Can you work these out from the model? Positions are in its coordinate system, mm. Face numbers are marked on the shaded views. A direction names the side the tool comes from. Give positions to 0.01 mm unless a question says otherwise; leave off trailing zeros. Write each loop counter-clockwise with the first axis right and the second up, starting at its lowest first coordinate (ties: lowest second). Pieces come first, ordered by that corner, then holes.
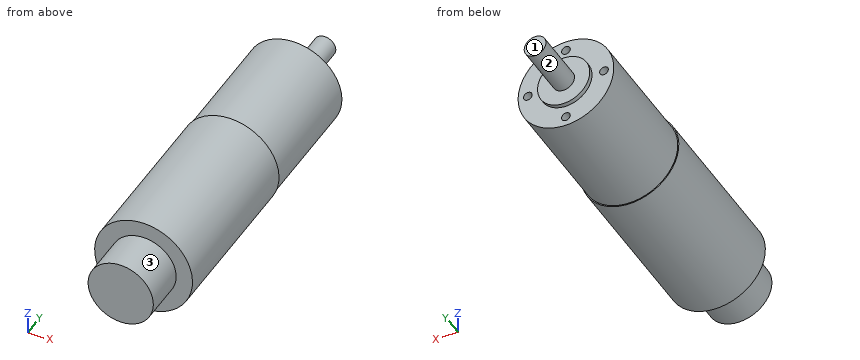
from build123d import *

# Parameters (mm, degrees)
SKETCH1_R           = 22.5
BOSS_EXTRUDE1_DEPTH = 75.7
SKETCH2_R           = 22
BOSS_EXTRUDE3_DEPTH = 56
SKETCH3_R           = 5
BOSS_EXTRUDE4_DEPTH = 27
SKETCH5_R           = 2
CUT_EXTRUDE2_DEPTH  = 9
CIRPATTERN1_COUNT   = 4
SKETCH6_R           = 12
BOSS_EXTRUDE5_DEPTH = 2
SKETCH7_R           = 15
BOSS_EXTRUDE6_DEPTH = 20


with BuildPart() as part:
    # Sketch1 → Boss-Extrude1 (new body)
    with BuildSketch(Plane(origin=(0, 0, 0), x_dir=(1, 0, 0), z_dir=(0, 1, 0))):
        with Locations(Location((0, 0, 0), (0, 0, 270))):
            Circle(SKETCH1_R)
    extrude(amount=BOSS_EXTRUDE1_DEPTH)

    # Sketch2 → Boss-Extrude3 (add)
    with BuildSketch(Plane(origin=(0, 75.7, 0), x_dir=(1, 0, 0), z_dir=(0, 1, 0))):
        with Locations(Location((0, 0, 0), (0, 0, 270))):
            Circle(SKETCH2_R)
    extrude(amount=BOSS_EXTRUDE3_DEPTH)

    # Sketch3 → Boss-Extrude4 (add)
    with BuildSketch(Plane(origin=(0, 131.7, 0), x_dir=(1, 0, 0), z_dir=(0, 1, 0))):
        with Locations(Location((0, 0, 0), (0, 0, 270))):
            Circle(SKETCH3_R)
    extrude(amount=BOSS_EXTRUDE4_DEPTH)

    # Sketch5 → Cut-Extrude2 (cut)
    with BuildSketch(Plane(origin=(0, 131.7, 0), x_dir=(1, 0, 0), z_dir=(0, 1, 0))):
        with Locations(Location((0, 17.5, 0), (0, 0, 270))):
            Circle(SKETCH5_R)
    cut_extrude2 = extrude(amount=-CUT_EXTRUDE2_DEPTH, mode=Mode.SUBTRACT)

    # CirPattern1: Cut-Extrude2 ×4 about axis
    cirpattern1_axis = Axis((0, 0, 0), (0, 1, 0))
    for i in range(1, CIRPATTERN1_COUNT):
        add(cut_extrude2.rotate(cirpattern1_axis, i * 360 / CIRPATTERN1_COUNT), mode=Mode.SUBTRACT)

    # Sketch6 → Boss-Extrude5 (add)
    with BuildSketch(Plane(origin=(0, 131.7, 0), x_dir=(1, 0, 0), z_dir=(0, 1, 0))):
        with Locations(Location((0, 0, 0), (0, 0, 270))):
            Circle(SKETCH6_R)
    extrude(amount=BOSS_EXTRUDE5_DEPTH)

    # Sketch7 → Boss-Extrude6 (add)
    with BuildSketch(Plane.XZ):
        with Locations(Location((0, 0, 0), (0, 0, 270))):
            Circle(SKETCH7_R)
    extrude(amount=BOSS_EXTRUDE6_DEPTH)


solid = part.part
(1) Imagine slicing it at D-D, the plane x = -10. Write out the boundary of the cut face in (y, z).
Returned:
outline: (-20, -11.18) - (0, -11.18) - (0, -20.16) - (75.7, -20.16) - (75.7, -19.6) - (131.7, -19.6) - (131.7, -6.63) - (133.7, -6.63) - (133.7, 6.63) - (131.7, 6.63) - (131.7, 19.6) - (75.7, 19.6) - (75.7, 20.16) - (0, 20.16) - (0, 11.18) - (-20, 11.18) - close
(2) Imagine slicing it at B-B, the plane x = 0. Write out the boundary of the cut face in (y, z), plus the area to 3 significant figures.
Returned:
outline: (-20, -15) - (0, -15) - (0, -22.5) - (75.7, -22.5) - (75.7, -22) - (131.7, -22) - (131.7, -19.5) - (122.7, -19.5) - (122.7, -15.5) - (131.7, -15.5) - (131.7, -12) - (133.7, -12) - (133.7, -5) - (158.7, -5) - (158.7, 5) - (133.7, 5) - (133.7, 12) - (131.7, 12) - (131.7, 15.5) - (122.7, 15.5) - (122.7, 19.5) - (131.7, 19.5) - (131.7, 22) - (75.7, 22) - (75.7, 22.5) - (0, 22.5) - (0, 15) - (-20, 15) - close
area: 6,700 mm2
(3) If I drill on L1, parallel to Y at x = -7, z = 14; L2, parallel to Y at x = -10, z = -7; L3, parallel to X at y = 127, z = 17.5, over which ranges is the centre line in solid material (lowest first)?
Returned:
L1: y = 0 to 131.7
L2: y = -20 to 131.7
L3: x = -13.33 to -2, 2 to 13.33
(4) Imagine slicing it at C-C, the plane y = 118. Write out the boundary of the cut face in (x, z).
Returned:
outline: circle Ø44 at (0, 0)
(5) Will these pins go through, and if not, where does the flat tip stop? P1, Ø1.2, axis at x = 18.5, z = 0, coming from the +Y side; P2, Ø4.5, axis at x = 17.5, z = 0, coming from the -Y side; P3, Ø2, axis at x = -15.5, z = -13, coming from the +Y side.
Returned:
P1: stops at y = 122.7
P2: stops at y = 0
P3: stops at y = 131.7
(6) Imagine slicing it at A-A, the plane z = 0. Write out the boundary of the cut face in (x, y).
Returned:
outline: (-22.5, 0) - (-15, 0) - (-15, -20) - (15, -20) - (15, 0) - (22.5, 0) - (22.5, 75.7) - (22, 75.7) - (22, 131.7) - (19.5, 131.7) - (19.5, 122.7) - (15.5, 122.7) - (15.5, 131.7) - (12, 131.7) - (12, 133.7) - (5, 133.7) - (5, 158.7) - (-5, 158.7) - (-5, 133.7) - (-12, 133.7) - (-12, 131.7) - (-15.5, 131.7) - (-15.5, 122.7) - (-19.5, 122.7) - (-19.5, 131.7) - (-22, 131.7) - (-22, 75.7) - (-22.5, 75.7) - close
(7) For the marked faces 1, 2 and 3, which set-ups out of +Z, -Z, +X, -X, +Y, -Y let a thin tool reach every point of the face, with its end or its side?
Returned:
face 1: +Z, -Z, +X, -X, +Y
face 2: +Y
face 3: -Y
